Read the model definition and answer for the solid it produces. Units are mm, in the model's axes. A direction names the side the tool comes from. Give positions to 0.01 mm unless a question says otherwise; leave off trailing zeros. Write each loop counter-clockwise with the first axis right and the second up, starting at its lowest first coordinate (ties: lowest second). Pieces come first, ordered by that corner, then holes. Notation, with made-up numbers: (46.25, -32.5) -> (52.25, -32.5) arc R24 ccw to (52.25, -4.5) -> close; hole circle Ø4 at (8, -29.5). An arc over 180 degrees is marked (long way). Use a Markdown table: item, result.
from build123d import *

# Parameters (mm, degrees)
SKETCH1_R               = 3.175
BOSS_EXTRUDE1_DEPTH     = 9.525
SKETCH2_R               = 3.175
BOSS_EXTRUDE2_DEPTH     = 12.7
CHAMFER1_SIZE           = 0.79375
CUT_EXTRUDE1_DEPTH      = 28.86051193
CUT_EXTRUDE1_DEPTH_BACK = 28.86051193
SKETCH3_W               = 9.525
SKETCH3_H               = 15.875
FILLET1_R               = 3.175


with BuildPart() as part:
    # Sketch1 → Boss-Extrude1 (new, symmetric)
    with BuildSketch(Plane(origin=(0, 0, 0), x_dir=(0, 0, -1), z_dir=(1, 0, 0))):
        with BuildLine():
            Line((-6.35, 0), (-6.35, -12.7))
            Line((-6.35, -12.7), (6.35, -12.7))
            Line((6.35, -12.7), (6.35, 0))
            ThreePointArc((6.35, 0), (0, 6.35), (-6.35, 0))
        make_face()
        with Locations(Location((0, 0, 0), (0, 0, 180))):
            Circle(SKETCH1_R, mode=Mode.SUBTRACT)
    extrude(amount=BOSS_EXTRUDE1_DEPTH, both=True)

    # Sketch2 → Boss-Extrude2 (add)
    with BuildSketch(Plane.XZ.offset(12.7)):
        with Locations(Location((0, 0, 0), (0, 0, 90))):
            Circle(SKETCH2_R)
    extrude(amount=BOSS_EXTRUDE2_DEPTH)

    # Chamfer1
    chamfer1_edges = [part.edges().sort_by_distance(p)[0] for p in [
        (0, -25.4, -3.175),
    ]]
    chamfer(chamfer1_edges, length=CHAMFER1_SIZE)

    # Sketch3 → Cut-Extrude1 (cut, two sides: drawn at the far end of the back side and taken through both)
    with BuildSketch(Plane.XY.offset(-CUT_EXTRUDE1_DEPTH_BACK)):
        with Locations((0, -1.5875)):
            Rectangle(SKETCH3_W, SKETCH3_H)
    extrude(amount=CUT_EXTRUDE1_DEPTH + CUT_EXTRUDE1_DEPTH_BACK, mode=Mode.SUBTRACT)

    # Fillet1
    fillet1_edges = [part.edges().sort_by_distance(p)[0] for p in [
        (-4.7625, -9.525, 0),
        (4.7625, -9.525, 0),
    ]]
    fillet(fillet1_edges, radius=FILLET1_R)


solid = part.part
Item 1: A cutting plane is placed at C-C (x = -8). Give the vertices of the cut face in (y, z) (3 decimals), then the cut area to 3 significant figures.
Return value:
| item | result |
|---|---|
| outline | (-12.7, -6.35) -> (0, -6.35) arc R6.35 ccw to (0, 6.35) -> (-12.7, 6.35) -> close; hole circle Ø6.35 at (0, 0) |
| area | 193 mm^2 |
Item 2: For a pull along Y with two mould halves and no side action, classify faces 1 (the face through (-4.762, -3, -2)), 2 (the face through (-7.2, 2.8, 1.5)), 3 (the face through (-7.11, 6.35, -0.14)), 4 (the face through (7.1, 2.8, 1.5)) as +Y half, -Y half, draft (parallel to the pull), parting line (faces both ways), or undercut.
Return value:
| item | result |
|---|---|
| face 1 | draft |
| face 2 | undercut |
| face 3 | +Y half |
| face 4 | undercut |
Item 3: A tool of negligible diameter and unlimited length cuts with its end or side. For faces 5 (the face through (9.525, -5, 0)), 6 (the face through (-3.86, -8.57, 0.09)), 7 (the face through (1.93, -18.57, -2.52)), from which of +Z, -Z, +X, -X, +Y, -Y can it reach the whole face along a straight path? Write none if from no direction.
Return value:
| item | result |
|---|---|
| face 5 | +Z, -Z, +X, +Y, -Y |
| face 6 | +Z, -Z, +Y |
| face 7 | -Y |
Item 4: Straight lines are drawn through the part: line 1 along Y through (x, z) = (-6.8, 0) (3 decimals); line 2 along X through (y, z) = (4, -0.25) (1 decimal); line 3 along Y through (x, z) = (-5.75, 2.5). For each, find the intervals that lie inside material, in ascending order. Write a range as [from, to].
Return value:
| item | result |
|---|---|
| line 1 | [-12.7, -3.175], [3.175, 6.35] |
| line 2 | [-9.5, -4.8], [4.8, 9.5] |
| line 3 | [-12.7, -1.96], [1.96, 5.84] |
Item 5: A cutting plane is placed at D-D (x = 0). Give the vertices of the cut face in (y, z) (3 decimals), then the cut area to 3 significant figures.
Return value:
| item | result |
|---|---|
| outline | (-25.4, -2.381) -> (-24.606, -3.175) -> (-12.7, -3.175) -> (-12.7, -6.35) -> (-9.525, -6.35) -> (-9.525, 6.35) -> (-12.7, 6.35) -> (-12.7, 3.175) -> (-24.606, 3.175) -> (-25.4, 2.381) -> close |
| area | 120 mm^2 |
Item 6: Each of these flat-tipped pins is pushed along its axis until it touches: P1, Ø1, axis at x = 0, z = -1, coming from the +Y side (3 decimals); P2, Ø4, axis at y = -21.5, z = 0.5, coming from the +X side (3 decimals). Where does it stop, or does it pass through?
Return value:
| item | result |
|---|---|
| P1 | y = -9.525 |
| P2 | x = 3.175 |
Item 7: A cutting plane is placed at B-B (z = 0). Count the separate pieces of the cut face and the enclosed holes in it, then the cut area to 3 significant figures.
Return value:
| item | result |
|---|---|
| separate pieces | 3 |
| enclosed holes | 0 |
| area | 236 mm^2 |
